Geometry: final body of the model. Coordinates: model frame, mm. Face numbers are marked on the shaded views. Coordinates: 2 decimals unless noted, no trailing zeros. Write each loop counter-clockwise with the first axis right and the second up, starting at its lowest first coordinate (ties: lowest second). Pieces come first, ordered by that corner, then holes. Notation, with made-up numbers: M -33.5,-13 L -6.5,-13 A23 ccw -6.5,25 Z; hole C 86.5,56.25 d2. An arc over 180 degrees is marked long. Write item = value, one per line. Start each with the question number.
Item 1: Pull-direction query (Y, two-part tool) for the marked faces 1, 2 and 3; classes: +Y half, -Y half, draft (parallel to the pull), parting line (faces both ways), or undercut.
Item 2: Section B-B on x = 4. Output: boundary loops of the cut face in (y, z), plus the area to 3 significant figures.
Item 3: Ray query, L1, parallel to Z at x = 1.75, y = 0; L2, parallel to Z at x = 5, y = 0; L3, parallel to Y at x = 4.5, z = 0. Return the intervals inside material, ascending. Write a range as [from, to].
Item 4: First-contact query: pin 1 Ø1.5 at (x, z) = (6, 1.5) entering from -Y; pin 2 Ø2 at (x, z) = (5.5, -2) entering from -Y; pin 3 Ø2 at (y, z) = (-0.5, 1) entering from -X. Flat tips, straight axial feed; report the tip coordinate or a pass-through.
Item 5: Section A-A on x = 1.25. Output: boundary loops of the cut face in (y, z), plus the area to 3 significant figures.
Autodesk Inventor part; units mm, degrees
ref_plane "Work Plane1" through (14.1836, 0, 0) normal (0, 0, 1) x (-1, 0, 0)
ref_plane "YZ Plane" through (0, 0, 0) normal (1, 0, 0) x (0, 1, 0)
ref_plane "XZ Plane" through (0, 0, 0) normal (0, 1, 0) x (-1, 0, 0)
sketch "Sketch1" plane through (0, 0, 0) normal (1, 0, 0) x (0, 1, 0)
  line L0 (-4.6188, 0) -> (-2.3094, 4)
  line L1 (-2.3094, 4) -> (2.3094, 4)
  line L2 (2.3094, 4) -> (4.6188, 0)
  line L3 (4.6188, 0) -> (2.3094, -4)
  line L4 (2.3094, -4) -> (-2.3094, -4)
  line L5 (-2.3094, -4) -> (-4.6188, 0)
  point P0 (0, 0)
  point P1 (0, 0)
  dimension "d0" = 9.2376
extrude "Body" add sketch "Sketch1" along normal blind 7.2
sketch "Sketch2" plane through (0, 0, 0) normal (-1, 0, 0) x (0, 0, 1)
  line L0 (0, -6.4663) -> (0, 6.4663)
  line L1 (-5.6, 0) -> (5.6, 0)
  point P0 (0, 0)
hole "Thread" at (0, 0, 0) direction (1, 0, 0) diameter 4.134 end through all
chamfer "Chamfer1" distance 0.433 angle 30 1 edges at (0, 0, -2.067) measured on face at (0, -2.8764, -1.7247)
chamfer "Chamfer2" distance 0.433 angle 30 1 edges at (7.2, 0, -2.067) measured on face at (7.2, -2.8764, -1.7247)
sketch "Sketch3" plane through (0, 0, 0) normal (0, 0, 1) x (1, 0, 0)
  line L0 (0, 2.3094) -> (0, 4.6188)
  line L1 (0, 4.6188) -> (7.2, 4.6188)
  line L2 (7.2, 2.3094) -> (7.2, 4.6188)
  line L3 (-1.44, 0) -> (8.64, 0)
  line L4 (0.3573, 4.6188) -> (0, 4)
  line L5 (7.2, 3.4) -> (4.811, 3.4)
  line L6 (4.811, 3.4) -> (2.7, 4.6188)
  dimension "d3" = 30
  dimension "d5" = 8
  dimension "d6" = 6.8
  dimension "d8" = 60
  dimension "d9" = 2.7
revolve "Chamfer3" cut sketch "Sketch3" angle 360 about axis through (-10, 0, 0) along (1, 0, 0)
ref_plane "Work Plane1" through (14.1836, 0, 0) normal (0, 0, 1) x (-1, 0, 0)
equation "\"d0\" = 1.1547 * SW"
equation "\"d1\" = KOH"
equation "\"d3\" = ANG1"
equation "\"d5\" = SW0"
equation "\"d6\" = SW1"
equation "\"d8\" = ANG2"
equation "\"d9\" = KOH1"
equation "\"d10\" = -0.5 * GD1 + 0.5 * NND"
equation "\"d39\" = -0.5 * GD1 + 0.5 * NND"
equation "\"d12\" = -0.5 * GD1 + 0.5 * NND"
equation "\"d40\" = -0.5 * GD1 + 0.5 * NND"
equation "\"ANG1\" = 30deg"
equation "\"ANG2\" = 60deg"
equation "\"NND\" = 5"
equation "\"KOH\" = 7.2"
equation "\"SW\" = 8"
equation "\"SW0\" = SW"
equation "\"SW1\" = 0.85 * SW"
equation "\"KOH1\" = 2.7"
equation "\"GUL\" = 0.541266 * PTC"
equation "\"THREADDIA\" = 5"
equation "\"TOA\" = 30deg"
equation "\"PTC\" = 0.8"
equation "\"E0\" = 1.155 * SW"
equation "\"GAL\" = 0.541266 * PTC"
properties part number "ANSI B18.16.3M - Property Class 9 - Metric M5 x 0.8 Top Insert Type" material "Steel, Mild"
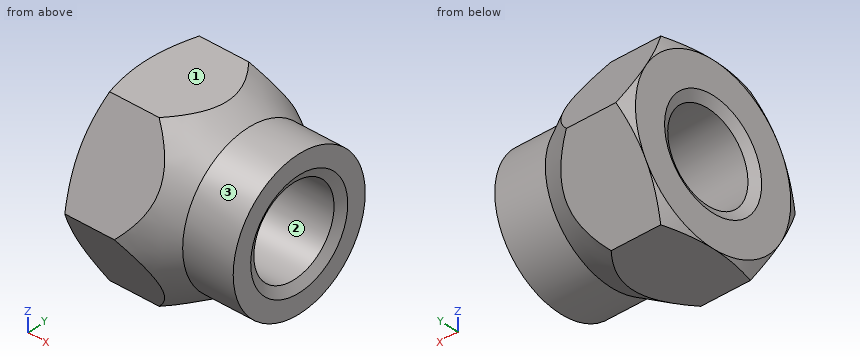
Responses:
q1.face_1 = draft
q1.face_2 = undercut
q1.face_3 = parting line
q2.outline = C 0,0 d7.74; hole C 0,0 d4.13
q2.area = 33.6 mm²
q3.L1 = [-4, -2.07], [2.07, 4]
q3.L2 = [-3.4, -2.07], [2.07, 3.4]
q3.L3 = [-3.58, -2.07], [2.07, 3.58]
q4.pin_1 = -3.32
q4.pin_2 = -3.25
q4.pin_3 = 0.22
q5.outline = M -4.62,0 L -2.31,-4 L 2.31,-4 L 4.62,0 L 2.31,4 L -2.31,4 Z; hole C 0,0 d4.13
q5.area = 42.0 mm²
